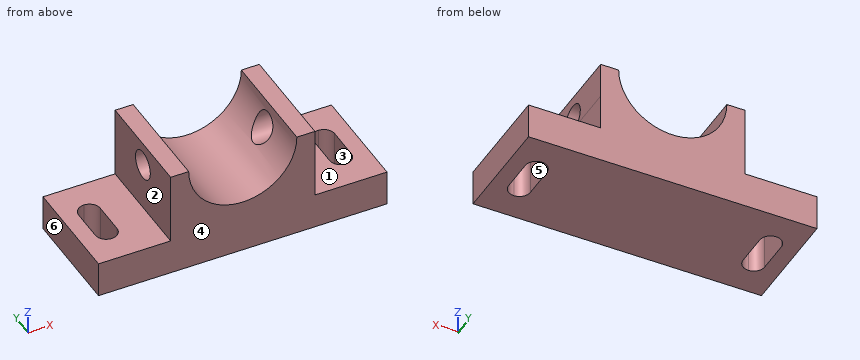
```python
from build123d import *

# Parameters (mm, degrees)
F1_DEPTH = 60
F2_R     = 8
F3_DEPTH = 120.001001
F6_DEPTH = 20.001


with BuildPart() as f1:
    # F0 (on Front) → F1 (new body)
    with BuildSketch(Plane.XZ):
        with BuildLine():
            Line((-80, 10), (-80, -10))
            Line((-80, -10), (80, -10))
            Line((80, -10), (80, 10))
            Line((80, 10), (40, 10))
            Line((40, 10), (40.000001, 30))
            Line((40.000001, 30), (40.000001, 50))
            Line((40.000001, 50), (30.000001, 50))
            ThreePointArc((30.000001, 50), (1e-06, 20), (-29.999999, 50))
            Line((-29.999999, 50), (-39.999999, 50))
            Line((-39.999999, 50), (-40, 10))
            Line((-40, 10), (-80, 10))
        make_face()
    extrude(amount=F1_DEPTH)

    # F2 (on face) → F3 (cut, through all)
    with BuildSketch(Plane(origin=(-40, 0, 1e-06), x_dir=(0, -1, 0), z_dir=(-1, 0, 0))):
        with Locations((30, 36.73611)):
            Circle(F2_R)
    extrude(amount=-F3_DEPTH, mode=Mode.SUBTRACT)

    # F4 (on face) + F5 (on face) → F6 (cut, through all)
    with BuildSketch(Plane.XY.offset(10)):
        with BuildLine():
            Line((-71, -21), (-71, -39))
            ThreePointArc((-71, -39), (-69.242641, -43.242641), (-65, -45))
            ThreePointArc((-65, -45), (-60.757359, -43.242641), (-59, -39))
            Line((-59, -39), (-59, -21))
            ThreePointArc((-59, -21), (-60.757359, -16.757359), (-65, -15))
            ThreePointArc((-65, -15), (-69.242641, -16.757359), (-71, -21))
        make_face()
    with BuildSketch(Plane.XY.offset(10)):
        with BuildLine():
            Line((59, -21), (59, -39))
            ThreePointArc((59, -39), (60.757359, -43.242641), (65, -45))
            ThreePointArc((65, -45), (69.242641, -43.242641), (71, -39))
            Line((71, -39), (71, -21))
            ThreePointArc((71, -21), (69.242641, -16.757359), (65, -15))
            ThreePointArc((65, -15), (60.757359, -16.757359), (59, -21))
        make_face()
    extrude(amount=-F6_DEPTH, mode=Mode.SUBTRACT)


solid = f1.part
```
The listing builds one solid part. Answer for the finished solid, in the listing's coordinates (mm). Face numbers are marked on the shaded views. A direction names the side the tool comes from. Give positions to 0.01 mm unless a question says otherwise; leave off trailing zeros. Order: outer loops, then holes, each group sorted by start corner. A loop starts at its lowest first (then second) coordinate and runs counter-clockwise, first axis right, second up. Notation, with made-up numbers: (-10.5, 54) - (42.5, 54) arc R15 cw to (42.5, 83) - close; hole circle Ø7 at (-8.75, -34.75). An arc over 180 degrees is marked (long way). Answer in a Markdown table with one row per item. Add a question column.
Q1. The part is cut by section C-C (y = -3.5). Determine the outline of the cut face in (x, z).
Q2. Find the intervals of material crossed by line 1 along X through (y, z) = (-22.5, 7.5); line 2 along Z through (x, y) = (35, -30); line 3 along X through (y, z) = (-41.5, 14), in increasing order. Write a range as [from, to].
Q3. The part is cut by section D-D (x = -69). Determine the outline of the cut face in (y, z).
Q4. The part is cut by section A-A (z = 2). Determine the outline of the cut face in (x, y).
Q5. For a pull along X with two mould halves and no side action, classify the marked faces 4, 5 and 6 as released by +X, released by -X, zero draft, split by the parting line, or undercut.
Q6. Which of the six approach directions +Z, -Z, +X, -X, +Y, -Y give full straight-line access (tool end or side, diameter ignored) to the marked faces 1, 2 and 3?
Q7. Given P1, Ø21, axis at y = -30, z = 36.74, coming from the +X side; P2, Ø5, axis at x = -52.5, y = -50.5, coming from the +Z side; P3, Ø1, axis at y = -36.5, z = 36, coming from the +X side; P4, Ø10, axis at x = 6, y = -52.5, coming from the +Z side, each flat-ended and moving along its own axis, determine where each tip first touches the part or whether it passes through.
Q8. The part is cut by section B-B (y = -29.5). Determine the outline of the cut face in (x, z).
Determined:
| question | item | result |
|---|---|---|
| 1 | outline | (-80, -10) - (80, -10) - (80, 10) - (40, 10) - (40, 50) - (30, 50) arc R30 cw to (-30, 50) - (-40, 50) - (-40, 10) - (-80, 10) - close |
| 2 | line 1 | x = [-80, -71], [-59, 59], [71, 80] |
| 2 | line 2 | z = [-10, 28.74], [44.74, 50] |
| 2 | line 3 | x = [-40, 40] |
| 3 | outline | (-60, -10) - (-43.47, -10) - (-43.47, 10) - (-60, 10) - close; (-16.53, -10) - (0, -10) - (0, 10) - (-16.53, 10) - close |
| 4 | outline | (-80, -60) - (80, -60) - (80, 0) - (-80, 0) - close; hole (-71, -39) arc R6 ccw to (-65, -45) arc R6 ccw to (-59, -39) - (-59, -21) arc R6 ccw to (-65, -15) arc R6 ccw to (-71, -21) - close; hole (59, -39) arc R6 ccw to (65, -45) arc R6 ccw to (71, -39) - (71, -21) arc R6 ccw to (65, -15) arc R6 ccw to (59, -21) - close |
| 5 | face 4 | zero draft |
| 5 | face 5 | undercut |
| 5 | face 6 | released by -X |
| 6 | face 1 | +Z, +X, +Y, -Y |
| 6 | face 2 | +Z, -X, +Y, -Y |
| 6 | face 3 | +Z, -Z |
| 7 | P1 | stops at x = 40 |
| 7 | P2 | stops at z = 10 |
| 7 | P3 | passes through |
| 7 | P4 | stops at z = 22.09 |
| 8 | outline | (-80, -10) - (-71, -10) - (-71, 10) - (-80, 10) - close; (-59, -10) - (59, -10) - (59, 10) - (40, 10) - (40, 28.75) - (21.18, 28.75) arc R30 cw to (-21.18, 28.75) - (-40, 28.75) - (-40, 10) - (-59, 10) - close; (-40, 44.72) - (-29.53, 44.72) arc R30 cw to (-30, 50) - (-40, 50) - close; (29.53, 44.72) - (40, 44.72) - (40, 50) - (30, 50) arc R30 cw to start; (71, -10) - (80, -10) - (80, 10) - (71, 10) - close |
